from build123d import *

# Parameters (mm, degrees)
BOSS_EXTRUDE1_DEPTH = 69.453125
SKETCH3_R           = 6.05234375
BOSS_EXTRUDE2_DEPTH = 3.175


with BuildPart() as part:
    # Sketch2 → Boss-Extrude1 (new body)
    with BuildSketch(Plane.XY):
        Polygon((45.24375, -11.988978873), (-45.24375, -11.988978873), (-47.0296875, 10.236021127), (47.0296875, 10.236021127), align=None)
    extrude(amount=BOSS_EXTRUDE1_DEPTH)

    # Sketch3 → Boss-Extrude2 (add)
    with BuildSketch(Plane.XZ.offset(11.988978873)):
        with Locations((36.01640625, 10.42590625)):
            Circle(SKETCH3_R)
        with Locations((-36.01640625, 9.22734375)):
            Circle(SKETCH3_R)
        with Locations((-36.01640625, 57.24921875)):
            Circle(SKETCH3_R)
        with Locations((36.01640625, 58.44778125)):
            Circle(SKETCH3_R)
        with BuildLine():
            Line((23.893870965, 33.420622184), (23.893870965, 38.778434684))
            ThreePointArc((23.893870965, 38.778434684), (29.152464715, 44.037028434), (34.411058465, 38.778434684))
            Line((34.411058465, 38.778434684), (34.411058465, 33.420622184))
            ThreePointArc((34.411058465, 33.420622184), (29.152464715, 28.162028434), (23.893870965, 33.420622184))
        make_face()
        with BuildLine():
            Line((-33.180557656, 32.453258987), (-33.180557656, 37.811071487))
            ThreePointArc((-33.180557656, 37.811071487), (-27.921963906, 43.069665237), (-22.663370156, 37.811071487))
            Line((-22.663370156, 37.811071487), (-22.663370156, 32.453258987))
            ThreePointArc((-22.663370156, 32.453258987), (-27.921963906, 27.194665237), (-33.180557656, 32.453258987))
        make_face()
    extrude(amount=BOSS_EXTRUDE2_DEPTH)


solid = part.part
Build history of the part. All positions in model axes, mm. A direction names the side the tool comes from. Round coordinates to 2 decimals unless told otherwise and drop trailing zeros. Loops run counter-clockwise (first coordinate to the right, second up) from the corner with the lowest first, then second, coordinate; pieces in that order, holes last. Notation, with made-up numbers: (31, 0) -> (71, 0) arc R10 cw to (71, 7) -> close; hole circle Ø2 at (-6, 8.5). An arc over 180 degrees is marked (long way). Answer in a Markdown table with one row per item.
Item 1: Saw through at B-B (y = -13.5). Write the cut outline in (x, z).
Answers below:
| item | result |
|---|---|
| outline | circle Ø12.1 at (-36.02, 9.23); circle Ø12.1 at (-36.02, 57.25); (-33.18, 32.45) arc R5.26 ccw to (-22.66, 32.45) -> (-22.66, 37.81) arc R5.26 ccw to (-33.18, 37.81) -> close; (23.89, 33.42) arc R5.26 ccw to (34.41, 33.42) -> (34.41, 38.78) arc R5.26 ccw to (23.89, 38.78) -> close; circle Ø12.1 at (36.02, 10.43); circle Ø12.1 at (36.02, 58.45) |
Item 2: Saw through at D-D (z = 55.5). Write the cut outline in (x, y), and give its area (3 significant figures).
Answers below:
| item | result |
|---|---|
| outline | (-47.03, 10.24) -> (-45.24, -11.99) -> (-41.81, -11.99) -> (-41.81, -15.16) -> (-30.22, -15.16) -> (-30.22, -11.99) -> (30.73, -11.99) -> (30.73, -15.16) -> (41.3, -15.16) -> (41.3, -11.99) -> (45.24, -11.99) -> (47.03, 10.24) -> close |
| area | 2,120 mm² |
Item 3: Saw through at A-A (z = 36.5). Write the cut outline in (x, y), and give its area (3 significant figures).
Answers below:
| item | result |
|---|---|
| outline | (-47.03, 10.24) -> (-45.24, -11.99) -> (-33.18, -11.99) -> (-33.18, -15.16) -> (-22.66, -15.16) -> (-22.66, -11.99) -> (23.89, -11.99) -> (23.89, -15.16) -> (34.41, -15.16) -> (34.41, -11.99) -> (45.24, -11.99) -> (47.03, 10.24) -> close |
| area | 2,120 mm² |
Item 4: Pin check, flat tips, straight feed: pin 1 (2 mm diameter, centred on x = -21, y = 1, fed in from -Z); pin 2 (3 mm diameter, centred on y = -3.5, z = 11.5, fed in from +X); pin 3 (3.5 mm diameter, centred on y = -14, z = 36.5, fed in from -X); pin 4 (3.5 mm diameter, centred on y = -13, z = 37, fed in from +X). Stop position of each tip, or through.
Answers below:
| item | result |
|---|---|
| pin 1 | stops at z = 0 |
| pin 2 | stops at x = 46.05 |
| pin 3 | stops at x = -33.18 |
| pin 4 | stops at x = 45.3 |
Item 5: Drill centre lines: L1, parallel to Y at x = 0, z = 54; L2, parallel to X at y = -13, z = 8; L3, parallel to X at y = 9, z = 32.5. Where is each one in solid material? Low to high. Write a range as [from, to].
Answers below:
| item | result |
|---|---|
| L1 | y = [-11.99, 10.24] |
| L2 | x = [-41.94, -30.09], [30.47, 41.56] |
| L3 | x = [-46.93, 46.93] |
Item 6: Mould opens along X. For faces 1 (the flat face through (-28, -15.164, 35)), 2 (the flat face through (-33.181, -14, 35)), 3 (the cylindrical face through (29.037, -13.554, 44.036)), 4 (the flat face through (1, -11.989, 34)) say: +X half, -X half, draft (parallel to the pull), parting line (faces both ways), or undercut.
Answers below:
| item | result |
|---|---|
| face 1 | draft |
| face 2 | -X half |
| face 3 | undercut |
| face 4 | undercut |
Item 7: Saw through at C-C (x = -32). Write the cut outline in (y, z).
Answers below:
| item | result |
|---|---|
| outline | (-15.16, 4.7) -> (-11.99, 4.7) -> (-11.99, 0) -> (10.24, 0) -> (10.24, 69.45) -> (-11.99, 69.45) -> (-11.99, 61.78) -> (-15.16, 61.78) -> (-15.16, 52.72) -> (-11.99, 52.72) -> (-11.99, 41.13) -> (-15.16, 41.13) -> (-15.16, 29.13) -> (-11.99, 29.13) -> (-11.99, 13.75) -> (-15.16, 13.75) -> close |
Item 8: Which spindle directions (+Z, -Z, +X, -X, +Y, -Y) get a long thin tool onto all of the face, cutting with end or side? Do faces 5 (the flat face through (-22.663, -14, 35)), 6 (the cylindrical face through (-30.244, -13.554, 11.045)), 7 (the flat face through (34.411, -14, 36)). Say none if no direction does.
Answers below:
| item | result |
|---|---|
| face 5 | +Z, -Z, -Y |
| face 6 | -Y |
| face 7 | +X, -Y |
